from build123d import *

# Parameters (mm, degrees)
BOSS_EXTRUDE1_DEPTH                               = 6.35
TAP_DRILL_FOR_6_32_TAP1_AT_2_COUNT                = 2
TAP_DRILL_FOR_6_32_TAP1_AT_2_PITCH                = 9.525
SKETCH7_W                                         = 6.35
SKETCH7_H                                         = 1.5875
CUT_EXTRUDE1_DEPTH                                = 91.02678768
CSK_FOR_6_FLAT_HEAD_MACHINE_SCREW_100_D           = 3.7973
CSK_FOR_6_FLAT_HEAD_MACHINE_SCREW_100_CSINK_D     = 7.0866
CSK_FOR_6_FLAT_HEAD_MACHINE_SCREW_100_CSINK_ANGLE = 100


with BuildPart() as part:
    # Sketch1 → Boss-Extrude1 (new body)
    with BuildSketch(Plane.XY):
        Polygon((-57.694743879, -6.959212537), (-57.694743879, 6.959212537), (-82.55, 10.509963411), (-82.55, -10.509963411), align=None)
        Polygon((57.694743879, -9.525), (-57.694743879, -9.525), (-79.919743879, -12.7), (79.919743879, -12.7), align=None)
        Polygon((-57.694743879, -9.525), (-57.694743879, -6.959212537), (-82.55, -10.509963411), (-82.55, -11.1125), (-86.767756121, -11.1125), (-88.9, -11.417106268), (-88.9, -12.7), (-79.919743879, -12.7), align=None)
        Polygon((0, -1.282893732), (-8.980256121, 0), (-57.694743879, -6.959212537), (-57.694743879, -9.525), align=None)
        Polygon((0, 1.282893732), (-57.694743879, 9.525), (-57.694743879, 6.959212537), (-8.980256121, 0), align=None)
        Polygon((79.919743879, 12.7), (-79.919743879, 12.7), (-57.694743879, 9.525), (57.694743879, 9.525), align=None)
        Polygon((-79.919743879, 12.7), (-88.9, 12.7), (-88.9, 11.417106268), (-86.767756121, 11.1125), (-82.55, 11.1125), (-82.55, 10.509963411), (-57.694743879, 6.959212537), (-57.694743879, 9.525), align=None)
        Polygon((57.694743879, -6.959212537), (8.980256121, 0), (0, -1.282893732), (57.694743879, -9.525), align=None)
        Polygon((57.694743879, 6.959212537), (57.694743879, 9.525), (0, 1.282893732), (8.980256121, 0), align=None)
        Polygon((8.980256121, 0), (0, 1.282893732), (-8.980256121, 0), (0, -1.282893732), align=None)
        Polygon((82.55, -10.509963411), (57.694743879, -6.959212537), (57.694743879, -9.525), (79.919743879, -12.7), (88.9, -12.7), (88.9, -11.417106268), (86.767756121, -11.1125), (82.55, -11.1125), align=None)
        Polygon((88.9, 12.7), (79.919743879, 12.7), (57.694743879, 9.525), (57.694743879, 6.959212537), (82.55, 10.509963411), (82.55, 11.1125), (86.767756121, 11.1125), (88.9, 11.417106268), align=None)
        Polygon((88.9, 11.1125), (88.9, 11.417106268), (86.767756121, 11.1125), align=None)
        Polygon((88.9, -11.1125), (86.767756121, -11.1125), (88.9, -11.417106268), align=None)
        Polygon((82.55, 10.509963411), (57.694743879, 6.959212537), (57.694743879, -6.959212537), (82.55, -10.509963411), align=None)
        Polygon((-88.9, -11.417106268), (-86.767756121, -11.1125), (-88.9, -11.1125), align=None)
        Polygon((-86.767756121, 11.1125), (-88.9, 11.417106268), (-88.9, 11.1125), align=None)
    extrude(amount=BOSS_EXTRUDE1_DEPTH)

    # Sketch4 → Tap Drill for #6-32 Tap1 (revolve, cut)
    with BuildSketch(Plane(origin=(-82.55, 4.7625, 3.175), x_dir=(0, 0, 1), z_dir=(0, 1, 0))):
        Polygon((0, 0), (0, 13.51269403), (1.35255, 12.7), (1.35255, 0), align=None)
    tap_drill_for_6_32_tap1 = revolve(axis=Axis((-88.9, 4.7625, 3.175), (1, 0, 0)), mode=Mode.SUBTRACT)

    # Tap Drill for #6-32 Tap1 at 2: Tap Drill for #6-32 Tap1 ×2
    with Locations(*[(0, -i * TAP_DRILL_FOR_6_32_TAP1_AT_2_PITCH, 0) for i in range(1, TAP_DRILL_FOR_6_32_TAP1_AT_2_COUNT)]):
        add(tap_drill_for_6_32_tap1, mode=Mode.SUBTRACT)

    # Mirror1: Tap Drill for #6-32 Tap1 across plane
    add(tap_drill_for_6_32_tap1.mirror(Plane(origin=(0, 0, 0), x_dir=(0, 0, 1), z_dir=(1, 0, 0))), mode=Mode.SUBTRACT)

    # Mirror1 copy 1 sketch → Mirror1 copy 1 (revolve, cut)
    with BuildSketch(Plane(origin=(82.55, -4.7625, 3.175), x_dir=(0, 0, 1), z_dir=(0, 1, 0))):
        Polygon((0, 0), (0, -13.51269403), (1.35255, -12.7), (1.35255, 0), align=None)
    revolve(axis=Axis((88.9, -4.7625, 3.175), (1, 0, 0)), mode=Mode.SUBTRACT)

    # Sketch5 → Tap Drill for #6-32 Tap2 (revolve, cut)
    with BuildSketch(Plane(origin=(-73.289583418, 12.7, 3.175), x_dir=(0, 0, 1), z_dir=(1, 0, 0))):
        Polygon((0, 0), (0, 7.16269403), (1.35255, 6.35), (1.35255, 0), align=None)
    tap_drill_for_6_32_tap2 = revolve(axis=Axis((-73.289583418, 19.05, 3.175), (0, -1, 0)), mode=Mode.SUBTRACT)

    # Mirror2: Tap Drill for #6-32 Tap2 across plane
    add(tap_drill_for_6_32_tap2.mirror(Plane(origin=(0, 0, 0), x_dir=(0, 0, 1), z_dir=(1, 0, 0))), mode=Mode.SUBTRACT)

    # Mirror3: Tap Drill for #6-32 Tap2 across plane
    add(tap_drill_for_6_32_tap2.mirror(Plane(origin=(0, 0, 0), x_dir=(0, 0, 1), z_dir=(0, -1, 0))), mode=Mode.SUBTRACT)

    # Mirror3 copy 1 sketch → Mirror3 copy 1 (revolve, cut)
    with BuildSketch(Plane(origin=(73.289583418, -12.7, 3.175), x_dir=(0, 0, 1), z_dir=(-1, 0, 0))):
        Polygon((0, 0), (0, 7.16269403), (1.35255, 6.35), (1.35255, 0), align=None)
    revolve(axis=Axis((73.289583418, -19.05, 3.175), (0, 1, 0)), mode=Mode.SUBTRACT)

    # Sketch7 → Cut-Extrude1 (cut, through all)
    with BuildSketch(Plane.XY.offset(6.35)):
        with Locations((-61.595, 11.90625)):
            Rectangle(SKETCH7_W, SKETCH7_H)
        with Locations((-61.595, -11.90625)):
            Rectangle(SKETCH7_W, SKETCH7_H)
        with Locations((61.595, -11.90625)):
            Rectangle(SKETCH7_W, SKETCH7_H)
        with Locations((61.595, 11.90625)):
            Rectangle(SKETCH7_W, SKETCH7_H)
    extrude(amount=-CUT_EXTRUDE1_DEPTH, mode=Mode.SUBTRACT)

    # CSK for #6 Flat Head Machine Screw (100)1 (through all)
    with Locations(Plane.XY.offset(6.35)):
        with Locations((-61.595, 4.7625), (-61.595, -4.7625), (61.595, -4.7625), (61.595, 4.7625)):
            CounterSinkHole(CSK_FOR_6_FLAT_HEAD_MACHINE_SCREW_100_D / 2, CSK_FOR_6_FLAT_HEAD_MACHINE_SCREW_100_CSINK_D / 2, counter_sink_angle=CSK_FOR_6_FLAT_HEAD_MACHINE_SCREW_100_CSINK_ANGLE)


solid = part.part
For this review, take the finished solid that the model builds, in its own axes (mm). A direction names the side the tool comes from. Round coordinates to 2 decimals unless told otherwise and drop trailing zeros. Loops run counter-clockwise (first coordinate to the right, second up) from the corner with the lowest first, then second, coordinate; pieces in that order, holes last. Notation, with made-up numbers: (50, 57) - (75, 57) arc R19 cw to (75, 63) - close; hole circle Ø4 at (22, -29). An arc over 180 degrees is marked (long way). One line per item, written item: value. Start each with the question number.
Item 1: For L1, parallel to Y at x = -3.5, z = 1 (3 decimals); L2, parallel to Y at x = 48, z = 1 (3 decimals); L3, parallel to Y at x = -44, z = 5.5 (3 decimals), list the stretches that pass through material, from the lowest coordinate up.
Item 2: Take a section at B-B (x = 76.5). State how many separate pieces and enclosed holes the cut face has, plus the area to 3 significant figures.
Item 3: For faces 1 (the flat face through (62, -11.112, 3)), 2 (the flat face through (-62, 11.112, 3)), 3 (the cylindrical face through (-74.63, -9.57, 3)), list the 3-axis set-ups (+Z, -Z, +X, -X, +Y, -Y) from which the entire face can be reached by the end or side of a thin tool; tool diameter is ignored.
Item 4: Take a section at A-A (x = -46.5). Give the boundary of the cut face in (y, z) (3 decimals).
Item 5: Clearance check with flat-ended pins moving along their axes: pin 1 Ø2.5 at (y, z) = (-4.76, 3.18) entering from +X; pin 2 Ø1 at (y, z) = (10, 5.5) entering from +X; pin 3 Ø3 at (y, z) = (-2, 3) entering from -X. State where each tip first meets the part, or that it passes through.
Item 6: The part is to be moulded in two halves that separate along Z. For faces 4 (the flat face through (-1, 9.525, 3)), 5 (the conical face through (69.18, -5, 3.14)), say which applies: +Z half, -Z half, draft (parallel to the pull), parting line (faces both ways), or undercut.
Answer below:
1. L1: y = -12.7 to -9.525, -1.783 to 1.783, 9.525 to 12.7
1. L2: y = -12.7 to -9.525, -8.14 to -5.574, 5.574 to 8.14, 9.525 to 12.7
1. L3: y = -12.7 to -9.525, -7.569 to -5.003, 5.003 to 7.569, 9.525 to 12.7
2. separate pieces: 1
2. enclosed holes: 2
2. area: 150 mm2
3. face 1: +Z, -Z, -Y
3. face 2: +Z, -Z, +Y
3. face 3: -Y
4. outline: (-12.7, 0) - (-9.525, 0) - (-9.525, 6.35) - (-12.7, 6.35) - close; (-7.926, 0) - (-5.36, 0) - (-5.36, 6.35) - (-7.926, 6.35) - close; (5.36, 0) - (7.926, 0) - (7.926, 6.35) - (5.36, 6.35) - close; (9.525, 0) - (12.7, 0) - (12.7, 6.35) - (9.525, 6.35) - close
5. pin 1: stops at x = 69.79
5. pin 2: stops at x = 82.55
5. pin 3: stops at x = -82.55
6. face 4: draft
6. face 5: undercut
